```python
from build123d import *
from OCP.BRepFilletAPI import BRepFilletAPI_MakeChamfer

# Parameters (mm, degrees)
SKETCH2_R             = 2.75
BOSS_EXTRUDE1_DEPTH   = 10
BOSS_EXTRUDE1_2_DEPTH = 10
SKETCH3_W             = 10
SKETCH3_H             = 27
BOSS_EXTRUDE2_DEPTH   = 15
SKETCH4_W             = 54
SKETCH4_H             = 27
BOSS_EXTRUDE3_DEPTH   = 10
CHAMFER1_SIZE         = 20
CHAMFER1_SIZE2        = 11.547005384
FILLET1_R             = 10
BOSS_EXTRUDE4_DEPTH   = 54
FILLET2_R             = 20
BOSS_EXTRUDE5_DEPTH   = 27
FILLET3_R             = 10
SKETCH7_R             = 4
BOSS_EXTRUDE6_DEPTH   = 27
FILLET4_R             = 2


with BuildPart() as part:
    # Sketch2 → Boss-Extrude1 (new body)
    with BuildSketch(Plane.XY):
        Polygon((44, -75), (44, -102), (74.026339821, -102), (74.026339821, -55), (59.01316991, -55), (59, -75), align=None)
        with Locations((59, -90)):
            Circle(SKETCH2_R, mode=Mode.SUBTRACT)
        with Locations((69, -65)):
            Circle(SKETCH2_R, mode=Mode.SUBTRACT)
    extrude(amount=BOSS_EXTRUDE1_DEPTH)



with BuildPart() as body_2:
    # Sketch2 → Boss-Extrude1 2 (new body)
    with BuildSketch(Plane.XY):
        Polygon((-20, -55), (-20, -102), (10, -102), (10, -75), (0, -75), (0, -55), align=None)
        with Locations((-10, -65)):
            Circle(SKETCH2_R, mode=Mode.SUBTRACT)
        with Locations((-5, -90)):
            Circle(SKETCH2_R, mode=Mode.SUBTRACT)
    extrude(amount=BOSS_EXTRUDE1_2_DEPTH)


with BuildPart() as part_1:
    add(part.part)

    add(body_2.part)  # Boss-Extrude2 merges body 2
    # Sketch3 → Boss-Extrude2 (add)
    with BuildSketch(Plane.XY.offset(10)):
        with Locations((5, -88.5)):
            Rectangle(SKETCH3_W, SKETCH3_H)
        with Locations((49, -88.5)):
            Rectangle(SKETCH3_W, SKETCH3_H)
    extrude(amount=BOSS_EXTRUDE2_DEPTH)

    # Sketch4 → Boss-Extrude3 (add)
    with BuildSketch(Plane.XY.offset(25)):
        with Locations((27, -88.5)):
            Rectangle(SKETCH4_W, SKETCH4_H)
    extrude(amount=BOSS_EXTRUDE3_DEPTH)

    # Chamfer1: one chamfer whose edges measure the first distance from different faces: ONE call of the kernel's chamfer builder (chamfer() names one face for all edges)
    chamfer1_edges_1 = [part_1.edges().sort_by_distance(p)[0] for p in [
        (44, -88.5, 25),
    ]]
    chamfer1_side_1 = [part_1.faces().sort_by_distance(p)[0] for p in [
        (44, -88.5, 12.5),
    ]]
    chamfer1_edges_2 = [part_1.edges().sort_by_distance(p)[0] for p in [
        (10, -88.5, 25),
    ]]
    chamfer1_side_2 = [part_1.faces().sort_by_distance(p)[0] for p in [
        (10, -88.5, 12.5),
    ]]
    chamfer1 = BRepFilletAPI_MakeChamfer(part_1.part.solid().wrapped)
    for e in chamfer1_edges_1:
        chamfer1.Add(CHAMFER1_SIZE, CHAMFER1_SIZE2, e.wrapped, chamfer1_side_1[0].wrapped)  # the first distance lies on this face
    for e in chamfer1_edges_2:
        chamfer1.Add(CHAMFER1_SIZE, CHAMFER1_SIZE2, e.wrapped, chamfer1_side_2[0].wrapped)  # the first distance lies on this face
    add(Compound.cast(chamfer1.Shape()), mode=Mode.REPLACE)

    # Fillet1
    # the kernel refuses this fillet: 10 mm, written as the material it adds along each edge
    with BuildSketch(Plane(origin=(44, -102, 5), x_dir=(0, 0, -1), z_dir=(0, 1, 0))) as fillet1_piece_1:
        with BuildLine():
            CenterArc((FILLET1_R * 0.267949192431, FILLET1_R), FILLET1_R, 240, 30)
            Line((-FILLET1_R * 0.232050807569, FILLET1_R * 0.133974596216), (0, 0))
            Line((0, 0), (FILLET1_R * 0.267949192431, 0))
        make_face()
    extrude(amount=27)
    with BuildSketch(Plane(origin=(10, -102, 5), x_dir=(0, 0, -1), z_dir=(0, 1, 0))) as fillet1_piece_2:
        with BuildLine():
            CenterArc((FILLET1_R * 0.267949192431, -FILLET1_R), FILLET1_R, 90, 30)
            Line((-FILLET1_R * 0.232050807569, -FILLET1_R * 0.133974596216), (0, 0))
            Line((0, 0), (FILLET1_R * 0.267949192431, 0))
        make_face()
    extrude(amount=27)
    with BuildSketch(Plane(origin=(21.547005384, -102, 25), x_dir=(-0.500000000000001, 0, -0.866025403784438), z_dir=(0, 1, 0))) as fillet1_piece_3:
        with BuildLine():
            CenterArc((FILLET1_R * 0.57735026919, -FILLET1_R), FILLET1_R, 90, 60)
            Line((-FILLET1_R * 0.288675134595, -FILLET1_R * 0.5), (0, 0))
            Line((0, 0), (FILLET1_R * 0.57735026919, 0))
        make_face()
    extrude(amount=27)
    with BuildSketch(Plane(origin=(32.452994616, -102, 25), x_dir=(0.5000000000000013, 0, -0.866025403784438), z_dir=(0, 1, 0))) as fillet1_piece_4:
        with BuildLine():
            CenterArc((FILLET1_R * 0.57735026919, FILLET1_R), FILLET1_R, 210, 60)
            Line((-FILLET1_R * 0.288675134595, FILLET1_R * 0.5), (0, 0))
            Line((0, 0), (FILLET1_R * 0.57735026919, 0))
        make_face()
    extrude(amount=27)

    # Sketch5 → Boss-Extrude4 (add)
    with BuildSketch(Plane.ZY):
        with BuildLine():
            ThreePointArc((35, -78.77790147), (38.839091833, -78.571636186), (42.413977278, -79.986332451))
            Line((42.413977278, -79.986332451), (35, -75))
            Line((35, -75), (35, -78.77790147))
        make_face()
        with BuildLine():
            ThreePointArc((35, -96.130929705), (39.540098119, -96.194122408), (43.533263146, -94.032845631))
            ThreePointArc((43.533263146, -94.032845631), (45.645892631, -91.040634418), (46.39125548, -87.454415588))
            ThreePointArc((46.39125548, -87.454415588), (45.334947826, -83.223842115), (42.413977278, -79.986332451))
            ThreePointArc((42.413977278, -79.986332451), (38.839091833, -78.571636186), (35, -78.77790147))
            Line((35, -78.77790147), (35, -96.130929705))
        make_face()
        with BuildLine():
            ThreePointArc((35, -78.77790147), (28.39125548, -87.454415588), (35, -96.130929705))
            Line((35, -96.130929705), (35, -78.77790147))
        make_face()
        with BuildLine():
            Line((35, -102), (43.533263146, -94.032845631))
            ThreePointArc((43.533263146, -94.032845631), (39.540098119, -96.194122408), (35, -96.130929705))
            Line((35, -96.130929705), (35, -102))
        make_face()
    extrude(amount=-BOSS_EXTRUDE4_DEPTH)

    # Fillet2
    fillet2_edges = [part_1.edges().sort_by_distance(p)[0] for p in [
        (27, -102, 35),
        (27, -75, 35),
    ]]
    fillet(fillet2_edges, radius=FILLET2_R)

    # Sketch6 → Boss-Extrude5 (add)
    with BuildSketch(Plane.XZ.offset(102)):
        with BuildLine():
            Line((27, -20.005137591), (27, 24.994862409))
            ThreePointArc((27, 24.994862409), (22.461220804, 23.739984394), (19, 20.546994264))
            Line((19, 20.546994264), (19, -20.005137591))
            Line((19, -20.005137591), (27, -20.005137591))
        make_face()
        with BuildLine():
            ThreePointArc((35, 20.546994264), (31.538779196, 23.739984394), (27, 24.994862409))
            Line((27, 24.994862409), (27, -20.005137591))
            Line((27, -20.005137591), (35, -20.005137591))
            Line((35, -20.005137591), (35, 20.546994264))
        make_face()
    extrude(amount=-BOSS_EXTRUDE5_DEPTH)

    # Fillet3
    fillet3_edges = [part_1.edges().sort_by_distance(p)[0] for p in [
        (27, -102, -20.005137591),
        (27, -75, -20.005137591),
    ]]
    fillet(fillet3_edges, radius=FILLET3_R)

    # Sketch7 → Boss-Extrude6 (add)
    with BuildSketch(Plane.XZ.offset(102)):
        with Locations((35, 20.546994264)):
            Circle(SKETCH7_R)
        with Locations((19, 20.546994264)):
            Circle(SKETCH7_R)
    extrude(amount=-BOSS_EXTRUDE6_DEPTH)

    # Fillet4
    # the kernel refuses this fillet: 2 mm, written as the material it adds along each edge
    with BuildSketch(Plane(origin=(19, -75, 16.546994264), x_dir=(-0.9855985596534884, 0, 0.16910197872576482), z_dir=(0, -1, 0))) as fillet4_piece_1:
        with BuildLine():
            CenterArc((1.691019787, 1.971197119), FILLET4_R, 189.735610317, 70.528779366)
            Line((-0.280177332, 1.632993162), (0, 0))
            ThreePointArc((0, 0), (0.676407915, 0.057605761), (1.35281583, 0))
        make_face()
    extrude(amount=27)
    with BuildSketch(Plane(origin=(16.982072855, -75, 17.093304927), x_dir=(0.9365633993502674, 0, -0.35049821539841175), z_dir=(0, -1, 0))) as fillet4_piece_2:
        with BuildLine():
            CenterArc((1.698511894, -1.970939444), FILLET4_R, 99.779167009, 70.738624206)
            Line((-0.274161714, -1.641456762), (0, 0))
            ThreePointArc((0, 0), (0.679404758, -0.058121111), (1.358809515, 0))
        make_face()
    extrude(amount=27)
    with BuildSketch(Plane(origin=(37.017927145, -75, 17.093304927), x_dir=(0.5000000000000021, 0, -0.8660254037844376), z_dir=(0, -1, 0))) as fillet4_piece_3:
        with BuildLine():
            CenterArc((1.664194985, -2), FILLET4_R, 90, 70.738624206)
            ThreePointArc((-0.223852102, -1.340243834), (-0.05459906, -0.679696867), (0, 0))
            Line((0, 0), (1.664194985, 0))
        make_face()
    extrude(amount=27)
    with BuildSketch(Plane(origin=(35, -75, 16.546994264), x_dir=(0, 0, -1), z_dir=(0, -1, 0))) as fillet4_piece_4:
        with BuildLine():
            CenterArc((1.656854249, 2), FILLET4_R, 199.471220634, 70.528779366)
            ThreePointArc((-0.228763834, 1.333333333), (-0.057605761, 0.676407915), (0, 0))
            Line((0, 0), (1.656854249, 0))
        make_face()
    extrude(amount=27)


solid = part_1.part
```
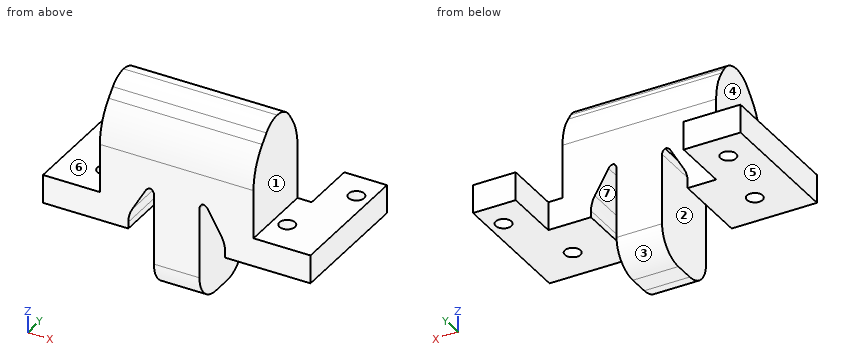
CAD build for the part. Positions are in the model's coordinates, mm. Face numbers are marked on the shaded views. A direction names the side the tool comes from. Give positions to 0.01 mm unless a question says otherwise; leave off trailing zeros. Write each loop counter-clockwise with the first axis right and the second up, starting at its lowest first coordinate (ties: lowest second). Pieces come first, ordered by that corner, then holes. Notation, with made-up numbers: (3.25, -35) -> (28.25, -35) arc R9 ccw to (28.25, -20) -> close; hole circle Ø3 at (62.5, 56.25). An arc over 180 degrees is marked (long way). Write each question's results on one line, items separated by ' | '.
1. Two-plate mould, pull along X, no slides. Class the marked faces 1, 2, 3 and 4: pulls with the +X half, pulls with the -X half, needs draft (parallel to the pull), parting line crosses it, or undercut.
Geometry check:
face 1: pulls with the +X half | face 2: undercut | face 3: needs draft | face 4: pulls with the -X half
2. Cut at B-B, the plane y = -90. Give the number of separate pieces and of enclosed holes in the cut face, then the cut area to 3 significant figures.
Geometry check:
separate pieces: 3 | enclosed holes: 0 | area: 2,880 mm²
3. Cut at D-D, the plane z = 26. Write the cut outline in (x, y), then the cut area to 3 significant figures.
Geometry check:
outline: (0, -102) -> (54, -102) -> (54, -75) -> (0, -75) -> close | area: 1,460 mm²
4. Wall check: probe 1 along Y at (x, z) = (-10, 3.5); probe 2 along Y at (x, z) = (-5, 3.75); probe 3 along Y at (x, z) = (15, 21). Give the ranges that are in metal, low to high. Write a range as [from, to].
Geometry check:
probe 1: [-102, -67.75], [-62.25, -55] | probe 2: [-102, -92.75], [-87.25, -55] | probe 3: [-102, -75]
5. Cut at C-C, the plane y = -65. Write the cut outline in (x, z), then the cut area to 3 significant figures.
Geometry check:
outline: (-20, 0) -> (-12.75, 0) -> (-12.75, 10) -> (-20, 10) -> close; (-7.25, 0) -> (0, 0) -> (0, 10) -> (-7.25, 10) -> close; (59.01, 0) -> (66.25, 0) -> (66.25, 10) -> (59.01, 10) -> close; (71.75, 0) -> (74.03, 0) -> (74.03, 10) -> (71.75, 10) -> close | area: 240 mm²
6. Drop flat-ended pins along their axis: P1, Ø6, axis at x = 59.5, y = -88, coming from the +Z side; P2, Ø9, axis at x = 0.5, y = -67, coming from the -Z side; P3, Ø21.5, axis at y = -84, z = 34, coming from the -X side; P4, Ø4.5, axis at x = 59, y = -90, coming from the -Z side. Give the stop position or say it passes through.
Geometry check:
P1: z = 10 | P2: z = 0 | P3: x = 0 | P4: through
7. Cut at A-A, the plane x = -5. Write the cut outline in (y, z).
Geometry check:
outline: (-102, 0) -> (-92.75, 0) -> (-92.75, 10) -> (-102, 10) -> close; (-87.25, 0) -> (-55, 0) -> (-55, 10) -> (-87.25, 10) -> close
8. Which spindle directions (+Z, -Z, +X, -X, +Y, -Y) get a long thin tool onto all of the face, cutting with end or side? Do the marked faces 5, 6 and 7. Say none if no direction does.
Geometry check:
face 5: -Z, -X, +Y, -Y | face 6: +Z, -X, +Y, -Y | face 7: -Z, +Y, -Y
